Verification items for the finished model (mm, model axes). Coordinates: 2 decimals unless noted, no trailing zeros. Write each loop counter-clockwise with the first axis right and the second up, starting at its lowest first coordinate (ties: lowest second). Pieces come first, ordered by that corner, then holes. Notation, with made-up numbers: (-22.5, 50.5) - (1.5, 50.5) arc R16 ccw to (1.5, 78.5) - close; hole circle Ø7 at (35.5, 52.5). An arc over 180 degrees is marked (long way). Use one line per item in the form item = value. Start each with the question number.
(1) Sectioned sample at A-A (y = 2). Record the cut outline in (x, z), and give its area (3 significant figures).
(2) Gauge pin test, flat ends, axial feed: pin 1 Ø8 at (x, z) = (-37.5, 7.5) entering from +Y; pin 2 Ø4 at (x, z) = (-22, -6.5) entering from +Y; pin 3 Ø2 at (x, z) = (-43.5, 7.5) entering from -Y. Record the tip position at first contact, or that the pin passes through.
(3) Material ranges on line 1 (Y direction, x = -15, z = -1.5); line 2 (X direction, y = 25.5, z = -9); line 3 (X direction, y = 28.5, z = -6.75), recorded low to high. Write a range as [from, to].
from build123d import *

# Parameters (mm, degrees)
SKETCH1_W           = 114.3
SKETCH1_H           = 25.4
BOSS_EXTRUDE1_DEPTH = 31.75
SKETCH2_RX          = 34.925
SKETCH2_RY          = 25.4
CUT_EXTRUDE1_DEPTH  = 71.138042459
FILLET1_R           = 2.54
FILLET2_R           = 22.86
FILLET3_R           = 10.16


with BuildPart() as part:
    # Sketch1 → Boss-Extrude1 (new body)
    with BuildSketch(Plane(origin=(0, 0, 0), x_dir=(1, 0, 0), z_dir=(0, 1, 0))):
        Rectangle(SKETCH1_W, SKETCH1_H)
    extrude(amount=BOSS_EXTRUDE1_DEPTH)

    # Sketch2 → Cut-Extrude1 (cut, through all)
    with BuildSketch(Plane.XY.offset(12.7)):
        with Locations(Location((-15.875, 31.75), (0, 0, 180))):
            Ellipse(SKETCH2_RX, SKETCH2_RY)
    extrude(amount=-CUT_EXTRUDE1_DEPTH, mode=Mode.SUBTRACT)

    # Fillet1
    fillet1_edges = [part.edges().sort_by_distance(p)[0] for p in [
        (-50.8, 31.75, 0),
    ]]
    fillet(fillet1_edges, radius=FILLET1_R)

    # Fillet2
    fillet2_edges = [part.edges().sort_by_distance(p)[0] for p in [
        (-57.15, 0, 0),
    ]]
    fillet(fillet2_edges, radius=FILLET2_R)

    # Fillet3
    fillet3_edges = [part.edges().sort_by_distance(p)[0] for p in [
        (57.15, 31.75, 0),
        (57.15, 0, 0),
    ]]
    fillet(fillet3_edges, radius=FILLET3_R)


solid = part.part
Answers below:
q1.outline = (-43.64, -12.7) - (53.04, -12.7) - (53.04, 12.7) - (-43.64, 12.7) - close
q1.area = 2,460 mm2
q2.pin_1 = 14.49
q2.pin_2 = 7.05
q2.pin_3 = 1.53
q3.line_1 = [0, 6.36]
q3.line_2 = [-57.15, -49.73], [17.98, 56.37]
q3.line_3 = [-57.15, -50.51], [18.76, 54.44]
